The model under review builds one solid part; all positions refer to its coordinate system, in mm. A direction names the side the tool comes from. Round coordinates to 2 decimals unless told otherwise and drop trailing zeros. Loops run counter-clockwise (first coordinate to the right, second up) from the corner with the lowest first, then second, coordinate; pieces in that order, holes last. Notation, with made-up numbers: (49.25, -18) -> (107.25, -18) arc R19 cw to (107.25, -8) -> close; hole circle Ø8 at (6, 53). An arc over 180 degrees is marked (long way). Write each question's results on one line, items separated by ' | '. Start each with the question number.
Item 1: Clearance check with flat-ended pins moving along their axes: pin 1 Ø5 at (x, z) = (56, -4.5) entering from +Y; pin 2 Ø5 at (y, z) = (16, -8) entering from +X; pin 3 Ø12 at (x, y) = (63, 8) entering from +Z. State where each tip first meets the part, or that it passes through.
Item 2: Tool access review of faces 1 (the cylindrical face through (61.445, 2.465, -20.979)), 2 (the flat face through (30, 5, 0)): name each direction out of +Z, -Z, +X, -X, +Y, -Y from which nothing blocks a thin tool from reaching the whole face with its end or side.
Item 3: We need section A-A (x = 33.25). Give the boundary of the cut face in (y, z).
Item 4: Mouldability with a two-part tool opening along X and no side actions: class faces 3 (the cylindrical face through (61.445, 2.465, 20.979)), 4 (the cylindrical face through (2.465, 42.165, -14.409)), 5 (the cylindrical face through (48.276, 2.465, 11.211)) as pulls with the +X half, pulls with the -X half, needs draft (parallel to the pull), parting line crosses it, or undercut.
Item 5: We need section D-D (y = 4). Give the number of separate pieces and of enclosed holes in the cut face, and give its area (3 significant figures).
Item 6: We need section C-C (z = 22.5). Give the boundary of the cut face in (x, y).
Item 7: For L1, parallel to Z at x = 33.25, y = 1.2; L2, parallel to Z at x = 46, y = 1; L3, parallel to X at y = 29, z = 21, list the stretches that pass through material, from the lowest coordinate up. Write a range as from..to.
Item 8: We need section B-B (y = 23). Give the boundary of the cut face in (x, z), and give its area (3 significant figures).
from build123d import *

# Parameters (mm, degrees)
SM_BASE_FLANGE_1_DEPTH  = 30
SKETCH_2_R              = 4.75
CUT_EXTRUDE_1_DEPTH     = 10
HOLE_WIZARD_1_OUTLINE_R = 1.6
HOLE_WIZARD_1_DEPTH     = 5
SKETCH_5_R              = 10
CUT_EXTRUDE_2_DEPTH     = 10
HOLE_WIZARD_2_OUTLINE_R = 1.6
HOLE_WIZARD_2_DEPTH     = 5
FILLET_1_R              = 30


# Read off the part's stored shape, not the designer's step: 孔1, 孔2
# Sheet-metal steps are written as plain solids
with BuildPart() as part:
    # Sketch 1 → 基体-法兰1 (new, symmetric)
    with BuildSketch(Plane.XY):
        with BuildLine():
            Line((70, 0), (5.7366, 0))
            ThreePointArc((5.7366, 0), (1.680211239, 1.680211239), (0, 5.7366))
            Line((0, 5.7366), (0, 60))
            Line((0, 60), (5, 60))
            Line((5, 60), (5, 5.7366))
            ThreePointArc((5, 5.7366), (5.215745145, 5.215745145), (5.7366, 5))
            Line((5.7366, 5), (70, 5))
            Line((70, 5), (70, 0))
        make_face()
    extrude(amount=SM_BASE_FLANGE_1_DEPTH, both=True)

    # Sketch 2 → 切除-拉伸1 (cut)
    with BuildSketch(Plane(origin=(0, 5, 0), x_dir=(1, 0, 0), z_dir=(0, 1, 0))):
        with Locations(Location((40, 0, 0), (0, 0, 180))):
            Circle(SKETCH_2_R)
    extrude(amount=-CUT_EXTRUDE_1_DEPTH, mode=Mode.SUBTRACT)

    # 孔1 outline → 孔1 (cut)
    with BuildSketch(Plane(origin=(0, 0, 0), x_dir=(1, 0, 0), z_dir=(0, 1, 0))):
        with Locations((33.25, -11.691342951)):
            Circle(HOLE_WIZARD_1_OUTLINE_R)
        with Locations((26.5, 0)):
            Circle(HOLE_WIZARD_1_OUTLINE_R)
        with Locations((33.25, 11.691342951)):
            Circle(HOLE_WIZARD_1_OUTLINE_R)
        with Locations((46.75, 11.691342951)):
            Circle(HOLE_WIZARD_1_OUTLINE_R)
        with Locations((53.5, 0)):
            Circle(HOLE_WIZARD_1_OUTLINE_R)
        with Locations((46.75, -11.691342951)):
            Circle(HOLE_WIZARD_1_OUTLINE_R)
    extrude(amount=HOLE_WIZARD_1_DEPTH, mode=Mode.SUBTRACT)

    # 草图5 → 切除-拉伸2 (cut)
    with BuildSketch(Plane.ZY):
        with Locations(Location((0, 30, 0), (0, 0, 270))):
            Circle(SKETCH_5_R)
    extrude(amount=-CUT_EXTRUDE_2_DEPTH, mode=Mode.SUBTRACT)

    # 孔2 outline → 孔2 (cut)
    with BuildSketch(Plane.YZ):
        with Locations((16.564971157, 13.435028843)):
            Circle(HOLE_WIZARD_2_OUTLINE_R)
        with Locations((16.564971157, -13.435028843)):
            Circle(HOLE_WIZARD_2_OUTLINE_R)
        with Locations((43.435028843, -13.435028843)):
            Circle(HOLE_WIZARD_2_OUTLINE_R)
        with Locations((43.435028843, 13.435028843)):
            Circle(HOLE_WIZARD_2_OUTLINE_R)
    extrude(amount=HOLE_WIZARD_2_DEPTH, mode=Mode.SUBTRACT)

    # 圆角1
    fillet_1_edges = [part.edges().sort_by_distance(p)[0] for p in [
        (70, 2.5, -30),
        (70, 2.5, 30),
        (2.5, 60, -30),
        (2.5, 60, 30),
    ]]
    fillet(fillet_1_edges, radius=FILLET_1_R - 0.0001)  # a hair under: the kernel refuses the full size


solid = part.part
Here are the results:
1) pin 1: stops at y = 5 | pin 2: stops at x = 5 | pin 3: stops at z = 24.15
2) face 1: -Z, +X, +Y, -Y | face 2: +Z, -Z, +X, +Y
3) outline: (0, -30) -> (5, -30) -> (5, -13.29) -> (0, -13.29) -> close; (0, -10.09) -> (5, -10.09) -> (5, 10.09) -> (0, 10.09) -> close; (0, 13.29) -> (5, 13.29) -> (5, 30) -> (0, 30) -> close
4) face 3: pulls with the +X half | face 4: needs draft | face 5: undercut
5) separate pieces: 1 | enclosed holes: 7 | area: 3,680 mm2
6) outline: (0, 5.74) arc R5.74 ccw to (5.74, 0) -> (59.84, 0) -> (59.84, 5) -> (5.74, 5) arc R0.74 cw to (5, 5.74) -> (5, 49.84) -> (0, 49.84) -> close
7) L1: z = -30..-13.29, -10.09..10.09, 13.29..30 | L2: z = -29.39..-13.1, -10.28..10.28, 13.1..29.39 | L3: x = 0..5
8) outline: (0, -30) -> (5, -30) -> (5, -7.14) -> (0, -7.14) -> close; (0, 7.14) -> (5, 7.14) -> (5, 30) -> (0, 30) -> close | area: 229 mm2
